Source: CAD feature listing. Evaluate the final solid. Frame: model axes, mm. A direction names the side the tool comes from. Round coordinates to 2 decimals unless told otherwise and drop trailing zeros. Write each loop counter-clockwise with the first axis right and the second up, starting at its lowest first coordinate (ties: lowest second). Pieces come first, ordered by that corner, then holes.
Solid Edge part; units mm, degrees
sketch "Sketch1" plane through (0, 0, 0) normal (0, 0, 1) x (1, 0, 0)
  circle A0 centre (0, 0) radius 2
extrude "Protrusion1" add sketch "Sketch1" along normal blind 20
sketch "Sketch2" plane through (0, 0, 20) normal (0, 0, 1) x (1, 0, 0)
  circle A0 centre (0, 0) radius 3
extrude "Top" add sketch "Sketch2" along normal blind 20
chamfer "Chamfer___Top" distance 1 angle 45 1 edges at (-3, 0, 40)
cosmetic_thread "Thread1"
properties material "Stainless Steel, 420"
1) Section query D-D on z = 5.5. Return the cut outline in (x, y), then the cut area to 3 significant figures.
Taken from the geometry:
outline: circle Ø4 at (0, 0)
area: 12.6 mm2
2) Section query C-C on z = 35.5. Return the cut outline in (x, y), then the cut area to 3 significant figures.
Taken from the geometry:
outline: circle Ø6 at (0, 0)
area: 28.3 mm2
3) Material intervals for line 1 (X direction, y = -0.05, z = 8); line 2 (X direction, y = -0.5, z = 29.5), sorted ascending.
Taken from the geometry:
line 1: x = -2 to 2
line 2: x = -2.96 to 2.96
4) Section query A-A on x = 0. Return the cut outline in (y, z), then the cut area to 3 significant figures.
Taken from the geometry:
outline: (-3, 20) - (-2, 20) - (-2, 0) - (2, 0) - (2, 20) - (3, 20) - (3, 39) - (2, 40) - (-2, 40) - (-3, 39) - close
area: 199 mm2
5) Contact query for flat-ended pins moving along their axis: P1, Ø1.5, axis at x = -1.5, z = 8, coming from the +Y side; P2, Ø1, axis at x = -1, z = 23.5, coming from the +Y side; P3, Ø2, axis at y = 2, z = 32, coming from the -X side. Output: stop coordinate, or through.
Taken from the geometry:
P1: stops at y = 1.85
P2: stops at y = 2.96
P3: stops at x = -2.83
6) Reachability of faces 1 (the face through (0, 0, 40)), 2 (the face through (0, 2, 10)) from +Z, -Z, +X, -X, +Y, -Y: full face, straight path, thin tool, end or side. Return the list, or none.
Taken from the geometry:
face 1: +Z, +X, -X, +Y, -Y
face 2: -Z
